```python
from build123d import *

# Parameters (mm, degrees)
SKETCH1_R           = 25.4
SKETCH1_R_2         = 5.08
SKETCH1_W           = 7.710600268
SKETCH1_H           = 7.62
BOSS_EXTRUDE1_DEPTH = 3.81


with BuildPart() as part:
    # Sketch1 → Boss-Extrude1 (new body)
    with BuildSketch(Plane.XY):
        with Locations(Location((0, 0, 0), (0, 0, 180))):
            Circle(SKETCH1_R)
        with Locations(Location((0, 16.51, 0), (0, 0, 180))):
            Circle(SKETCH1_R_2, mode=Mode.SUBTRACT)
        with Locations(Location((0, -16.51, 0), (0, 0, 180))):
            Circle(SKETCH1_R_2, mode=Mode.SUBTRACT)
        Rectangle(SKETCH1_W, SKETCH1_H, mode=Mode.SUBTRACT)
    extrude(amount=BOSS_EXTRUDE1_DEPTH)


solid = part.part
```
Read the model definition and answer for the solid it produces. Units are mm, in the model's axes. A direction names the side the tool comes from. Give positions to 0.01 mm unless a question says otherwise; leave off trailing zeros. Loops run counter-clockwise (first coordinate to the right, second up) from the corner with the lowest first, then second, coordinate; pieces in that order, holes last.
Item 1: The part is cut by section B-B (y = 0). Write down the section's boundary in (x, z).
Item 2: Each of these flat-tipped pins is pushed along its axis until it touches: pin 1 Ø1.1 at (y, z) = (1.5, 2.5) entering from +X; pin 2 Ø1.5 at (y, z) = (-9.5, 1.5) entering from +X; pin 3 Ø1.5 at (y, z) = (14, 2) entering from +X. Where does it stop, or does it pass through?
Item 3: The part is cut by section A-A (x = 0). Write down the section's boundary in (y, z).
Item 4: Find the intervals of material crossed by line 1 along Y through (x, z) = (0, 2.7); line 2 along X through (y, z) = (16.51, 1.85); line 3 along X through (y, z) = (2, 3.6), in increasing order.
Item 5: The part is cut by section C-C (z = 0.7). Write down the section's boundary in (x, y).
Item 6: The part is cut by section D-D (y = 18). Write down the section's boundary in (x, z), and give its area (3 significant figures).
Item 7: The mould has two halves that part along X. Classify faces 1 (the flat face through (0, 5, 0)), 2 (the cylindrical face through (0.661, -21.547, 1.878)), 3 (the cylindrical face through (-11.721, 22.534, 1.878)): released by +X, released by -X, zero draft, split by the parting line, or undercut.
Item 8: For faces 4 (the flat face through (0, 5, 3.81)), 5 (the flat face through (-3.855, 0, 2)), determine the directions among +Z, -Z, +X, -X, +Y, -Y from which every point of the face is accessible in a straight line to the end or side of a thin tool.
Taken from the geometry:
1. outline: (-25.4, 0) - (-3.86, 0) - (-3.86, 3.81) - (-25.4, 3.81) - close; (3.86, 0) - (25.4, 0) - (25.4, 3.81) - (3.86, 3.81) - close
2. pin 1: stops at x = 25.38
2. pin 2: stops at x = 23.85
2. pin 3: stops at x = 21.67
3. outline: (-25.4, 0) - (-21.59, 0) - (-21.59, 3.81) - (-25.4, 3.81) - close; (-11.43, 0) - (-3.81, 0) - (-3.81, 3.81) - (-11.43, 3.81) - close; (3.81, 0) - (11.43, 0) - (11.43, 3.81) - (3.81, 3.81) - close; (21.59, 0) - (25.4, 0) - (25.4, 3.81) - (21.59, 3.81) - close
4. line 1: y = -25.4 to -21.59, -11.43 to -3.81, 3.81 to 11.43, 21.59 to 25.4
4. line 2: x = -19.3 to -5.08, 5.08 to 19.3
4. line 3: x = -25.32 to -3.86, 3.86 to 25.32
5. outline: circle Ø50.8 at (0, 0); hole circle Ø10.16 at (0, -16.51); hole circle Ø10.16 at (0, 16.51); hole (-3.86, -3.81) - (3.86, -3.81) - (3.86, 3.81) - (-3.86, 3.81) - close
6. outline: (-17.92, 0) - (-4.86, 0) - (-4.86, 3.81) - (-17.92, 3.81) - close; (4.86, 0) - (17.92, 0) - (17.92, 3.81) - (4.86, 3.81) - close
6. area: 99.6 mm2
7. face 1: zero draft
7. face 2: undercut
7. face 3: split by the parting line
8. face 4: +Z, +X, -X, +Y, -Y
8. face 5: +Z, -Z
